Geometry: see drawing. Coordinates: mm, zero at the bounding-box minimum. A direction names the side the tool comes from. Coordinates: 2 decimals unless noted, no trailing zeros. Write each loop counter-clockwise with the first axis right and the second up, starting at its lowest first coordinate (ties: lowest second). Pieces come first, ordered by that corner, then holes. Notation, with made-up numbers: (47.25, 28) - (68.25, 28) arc R18 ccw to (68.25, 57) - close; hole circle Ø3 at (43, 35). An arc over 180 degrees is marked (long way). Use a Markdown table: item, result. Add a question column.
Q1. Pin query (flat end, axial travel): P1, Ø1, axis at x = 29.5, z = 30, coming from the -Y side; P2, Ø1, axis at y = 7, z = 29, coming from the +X side; P3, Ø10, axis at x = 10.5, y = 15, coming from the -Z side; P4, Ø6, axis at y = 9, z = 32, coming from the +X side. Return the tip coordinate at first contact, or that it passes through.
Q2. Section query C-C (y = 8.5). Return the cut outline in (x, z).
Q3. Section query A-A (x = 11). Return the cut outline in (y, z).
Q4. Set-up query: the marked faces 1, 2, 3 and 4. Return all of +Z, -Z, +X, -X, +Y, -Y with unobstructed straight access to the full face (end or side cutting, diameter ignored); none if empty.
Q5. Section query B-B (z = 32). Return the cut outline in (x, y).
Q6. Material intervals for probe 1 along Z at (x, y) = (11, 5.15); probe 2 along Y at (x, z) = (50, 35.5); probe 3 along Y at (x, z) = (6, 34), sorted ascending. Write a range as from..to.
Q7. Section query D-D (z = 27). Return the cut outline in (x, y).
Q8. Mould query, pull axis Z, two halves, no side actions, for the marked faces 5, 6 and 7. Classes: released by +Z, released by -Z, zero draft, split by the parting line, or undercut.
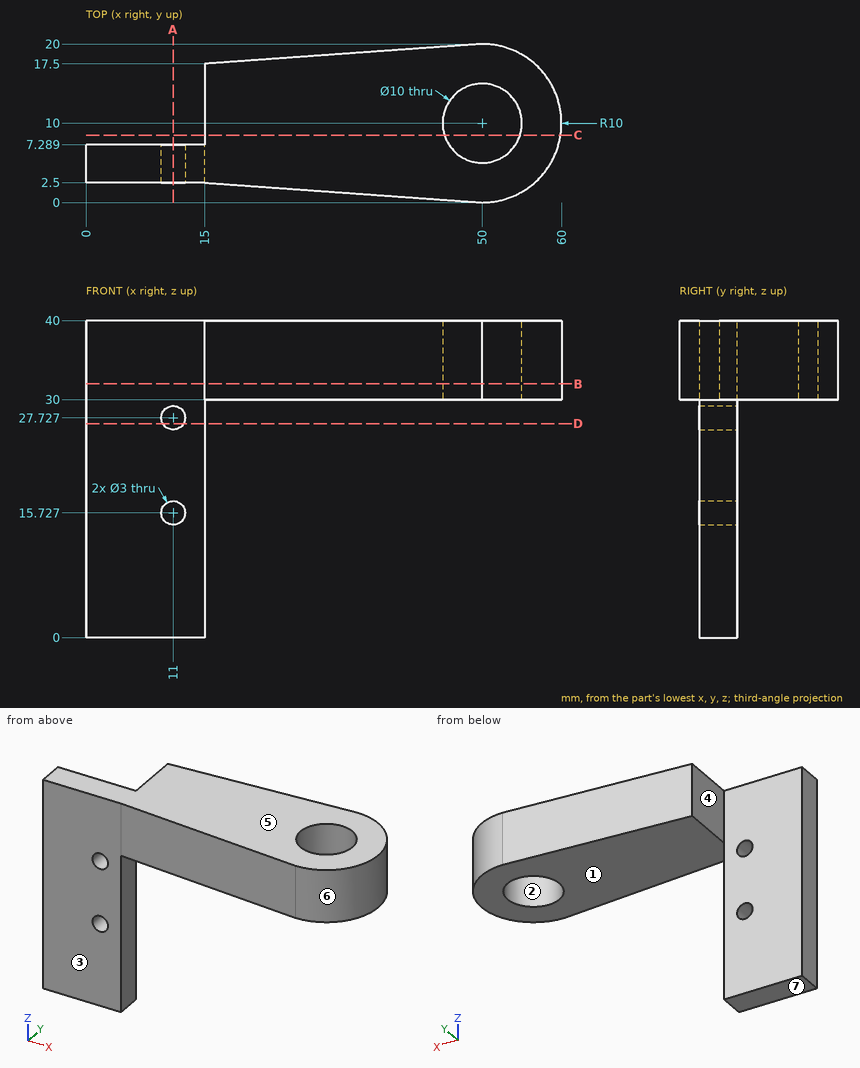
Values follow:
| question | item | result |
|---|---|---|
| 1 | P1 | y = 1.43 |
| 1 | P2 | x = 15 |
| 1 | P3 | z = 30 |
| 1 | P4 | x = 60 |
| 2 | outline | (15, 30) - (45.23, 30) - (45.23, 40) - (15, 40) - close; (54.77, 30) - (59.89, 30) - (59.89, 40) - (54.77, 40) - close |
| 3 | outline | (2.5, 0) - (7.29, 0) - (7.29, 14.23) - (2.5, 14.23) - close; (2.5, 17.23) - (7.29, 17.23) - (7.29, 26.23) - (2.5, 26.23) - close; (2.5, 29.23) - (7.29, 29.23) - (7.29, 40) - (2.5, 40) - close |
| 4 | face 1 | -Z, +X, +Y, -Y |
| 4 | face 2 | +Z, -Z |
| 4 | face 3 | +Z, -Z, -X, -Y |
| 4 | face 4 | +Z, -Z, -X, +Y |
| 5 | outline | (0, 2.5) - (15, 2.5) - (50, 0) arc R10 ccw to (50, 20) - (15, 17.5) - (15, 7.29) - (0, 7.29) - close; hole circle Ø10 at (50, 10) |
| 6 | probe 1 | 0..14.23, 17.23..26.23, 29.23..40 |
| 6 | probe 2 | 0..5, 15..20 |
| 6 | probe 3 | 2.5..7.29 |
| 7 | outline | (0, 2.5) - (9.69, 2.5) - (9.69, 7.29) - (0, 7.29) - close; (12.31, 2.5) - (15, 2.5) - (15, 7.29) - (12.31, 7.29) - close |
| 8 | face 5 | released by +Z |
| 8 | face 6 | zero draft |
| 8 | face 7 | released by -Z |
